Work out the finished part from the listing and answer in its coordinate system (mm). Coordinates: 2 decimals unless noted, no trailing zeros. Order: outer loops, then holes, each group sorted by start corner. A loop starts at its lowest first (then second) coordinate and runs counter-clockwise, first axis right, second up.
1. The part is cut by section D-D, the plane x = 13. Give the vertices of the cut face in (y, z).
2. The part is cut by section C-C, the plane z = 0.3. Count the separate pieces of the cut face and the enclosed holes in it, then the cut area to 3 significant figures.
3. Flat-ended cylindrical pins translate along their axes: pin 1 Ø0.5 at (x, z) = (-26, 0.5) entering from +Y; pin 2 Ø0.5 at (y, z) = (0, 0.5) entering from +X; pin 3 Ø3 at (x, y) = (13.97, -13.97) entering from -Z; pin 4 Ø0.5 at (x, z) = (25, 0.5) entering from +Y. Find the tip coordinate at first contact, or state that the pin passes through.
4. Find the intervals of material crossed by probe 1 along Y at (x, z) = (0, 0.7); probe 2 along Y at (x, z) = (20, 0.65); probe 3 along X at (y, z) = (19.5, 0.35) (3 decimals), in increasing order.
5. Determine the mould class of faces 1 (the cylindrical face through (-21.22, -20.85, 0.5)), 2 (the flat face through (0, -6, 0)), 3 (the cylindrical face through (-14.19, -12.28, 0.5)) for opening direction X: +X half, -X half, draft (parallel to the pull), parting line (faces both ways), or undercut.
6. The part is cut by section A-A, the plane y = 0. Give the vertices of the cut face in (x, z), then the cut area to 3 significant figures.
```python
from build123d import *

# Parameters (mm, degrees)
SKETCH1_R           = 1.7
SKETCH1_R_2         = 3
BOSS_EXTRUDE1_DEPTH = 1.016


with BuildPart() as part:
    # Sketch1 → Boss-Extrude1 (new body)
    with BuildSketch(Plane.XY):
        with BuildLine():
            Line((-29.326822194, 5), (-20.106608804, 5))
            ThreePointArc((-20.106608804, 5), (-19.399502023, 4.707106781), (-19.106608804, 4))
            Line((-19.106608804, 4), (-19.106608804, -4))
            ThreePointArc((-19.106608804, -4), (-19.399502023, -4.707106781), (-20.106608804, -5))
            Line((-20.106608804, -5), (-29.326822194, -5))
            ThreePointArc((-29.326822194, -5), (-21.03642674, -21.03642674), (-5, -29.326822194))
            Line((-5, -29.326822194), (-5, -20.106608804))
            ThreePointArc((-5, -20.106608804), (-4.707106781, -19.399502023), (-4, -19.106608804))
            Line((-4, -19.106608804), (4, -19.106608804))
            ThreePointArc((4, -19.106608804), (4.707106781, -19.399502023), (5, -20.106608804))
            Line((5, -20.106608804), (5, -29.326822194))
            ThreePointArc((5, -29.326822194), (21.03642674, -21.03642674), (29.326822194, -5))
            Line((29.326822194, -5), (20.106608804, -5))
            ThreePointArc((20.106608804, -5), (19.399502023, -4.707106781), (19.106608804, -4))
            Line((19.106608804, -4), (19.106608804, 4))
            ThreePointArc((19.106608804, 4), (19.399502023, 4.707106781), (20.106608804, 5))
            Line((20.106608804, 5), (29.326822194, 5))
            ThreePointArc((29.326822194, 5), (21.03642674, 21.03642674), (5, 29.326822194))
            Line((5, 29.326822194), (5, 20.106608804))
            ThreePointArc((5, 20.106608804), (4.707106781, 19.399502023), (4, 19.106608804))
            Line((4, 19.106608804), (-4, 19.106608804))
            ThreePointArc((-4, 19.106608804), (-4.707106781, 19.399502023), (-5, 20.106608804))
            Line((-5, 20.106608804), (-5, 29.326822194))
            ThreePointArc((-5, 29.326822194), (-21.03642674, 21.03642674), (-29.326822194, 5))
        make_face()
        with Locations((13.965358928, 13.965358928)):
            Circle(SKETCH1_R, mode=Mode.SUBTRACT)
        with Locations((13.965358928, -13.965358928)):
            Circle(SKETCH1_R, mode=Mode.SUBTRACT)
        with Locations((-13.965358928, -13.965358928)):
            Circle(SKETCH1_R, mode=Mode.SUBTRACT)
        with Locations((-13.965358928, 13.965358928)):
            Circle(SKETCH1_R, mode=Mode.SUBTRACT)
        Circle(SKETCH1_R_2, mode=Mode.SUBTRACT)
    extrude(amount=BOSS_EXTRUDE1_DEPTH)


solid = part.part
```
Geometry says:
1. outline: (-26.76, 0) - (-15.36, 0) - (-15.36, 1.02) - (-26.76, 1.02) - close; (-12.57, 0) - (12.57, 0) - (12.57, 1.02) - (-12.57, 1.02) - close; (15.36, 0) - (26.76, 0) - (26.76, 1.02) - (15.36, 1.02) - close
2. separate pieces: 1
2. enclosed holes: 5
2. area: 2,300 mm2
3. pin 1: stops at y = 14.9
3. pin 2: stops at x = 19.11
3. pin 3: passes through
3. pin 4: stops at y = 16.51
4. probe 1: y = -19.11 to -3, 3 to 19.11
4. probe 2: y = -22.02 to -4.99, 4.99 to 22.02
4. probe 3: x = -22.468 to -4.795, 4.795 to 22.468
5. face 1: -X half
5. face 2: draft
5. face 3: undercut
6. outline: (-19.11, 0) - (-3, 0) - (-3, 1.02) - (-19.11, 1.02) - close; (3, 0) - (19.11, 0) - (19.11, 1.02) - (3, 1.02) - close
6. area: 32.7 mm2
